Work out the finished part from the listing and answer in its coordinate system (mm). Face numbers are marked on the shaded views. A direction names the side the tool comes from. Give positions to 0.01 mm unless a question says otherwise; leave off trailing zeros. Loops run counter-clockwise (first coordinate to the right, second up) from the corner with the lowest first, then second, coordinate; pieces in that order, holes last. Notation, with made-up numbers: M -25.5,-35 L 29.5,-35 A25 ccw 29.5,-14 Z; hole C 2.25,-40 d9. An arc over 180 degrees is marked long. Use a Markdown table: item, result.
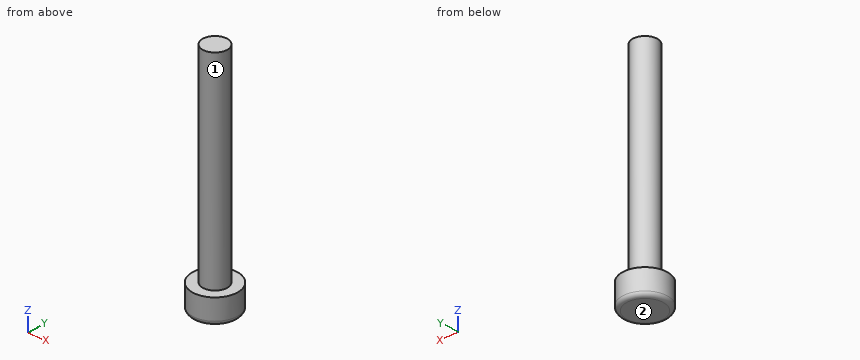
```python
from build123d import *

# Parameters (mm, degrees)
SKETCH_2_R      = 2.75
EXTRUDE_1_DEPTH = 3
SKETCH_3_R      = 1.5
EXTRUDE_2_DEPTH = 25
FILLET_1_R      = 0.5


with BuildPart() as part:
    # ｽｹｯﾁ2 → ﾎﾞｽ - 押し出し1 (new body)
    with BuildSketch(Plane.XY):
        Circle(SKETCH_2_R)
    extrude(amount=EXTRUDE_1_DEPTH)

    # ｽｹｯﾁ3 → ﾎﾞｽ - 押し出し2 (add)
    with BuildSketch(Plane.XY.offset(3)):
        Circle(SKETCH_3_R)
    extrude(amount=EXTRUDE_2_DEPTH)

    # ﾌｨﾚｯﾄ1
    fillet_1_edges = [part.edges().sort_by_distance(p)[0] for p in [
        (-2.75, 0, 0),
    ]]
    fillet(fillet_1_edges, radius=FILLET_1_R)


solid = part.part
```
(1) Consider probe 1 along Z at (x, y) = (-0.2, -1.75); probe 2 along X at (y, z) = (-0.15, 2); probe 3 along Y at (x, z) = (0, 25.75). Determine where each line is inside the solid, lowest interval first. Write a range as [from, to].
Entries:
| item | result |
|---|---|
| probe 1 | z = [0, 3] |
| probe 2 | x = [-2.75, 2.75] |
| probe 3 | y = [-1.5, 1.5] |
(2) Which of the six approach directions +Z, -Z, +X, -X, +Y, -Y give full straight-line access (tool end or side, diameter ignored) to the marked faces 1 and 2?
Entries:
| item | result |
|---|---|
| face 1 | +Z |
| face 2 | -Z, +X, -X, +Y, -Y |
(3) Given P1, Ø3, axis at x = 2, z = 14.5, coming from the +Y side; P2, Ø1, axis at y = -0.5, z = 19.5, coming from the -X side, each flat-ended and moving along its own axis, determine where each tip first touches the part or whether it passes through.
Entries:
| item | result |
|---|---|
| P1 | stops at y = 1.41 |
| P2 | stops at x = -1.5 |
(4) A cutting plane is placed at C-C (z = 9.75). Write down the section's boundary in (x, y).
Entries:
| item | result |
|---|---|
| outline | C 0,0 d3 |
(5) A cutting plane is placed at A-A (x = 0). Write down the section's boundary in (y, z), and give its area (3 significant figures).
Entries:
| item | result |
|---|---|
| outline | M -2.75,0.5 A0.5 ccw -2.25,0 L 2.25,0 A0.5 ccw 2.75,0.5 L 2.75,3 L 1.5,3 L 1.5,28 L -1.5,28 L -1.5,3 L -2.75,3 Z |
| area | 91.4 mm² |
